Here's how the part is built. I have some questions about the finished solid (model axes, mm). A direction names the side the tool comes from. Coordinates: 2 decimals unless noted, no trailing zeros. Loops run counter-clockwise (first coordinate to the right, second up) from the corner with the lowest first, then second, coordinate; pieces in that order, holes last. Notation, with made-up numbers: (-18.5, -2.5) -> (34.5, -2.5) arc R23 ccw to (34.5, 7.5) -> close; hole circle Ø1 at (24.25, 3). An arc over 180 degrees is marked (long way). Answer as a JSON object with one key per item and string values. Group by question number.
1) Which directions (+Z, -Z, +X, -X, +Y, -Y) give clear straight access to the entire face, cutting with the end or side of a thin tool? Please do faces 4 (the flat face through (2, 141, 17)), 5 (the flat face through (-2, 278, 0)).
2) I want a section at A-A (z = 6.5). Write out the boundary of the cut face in (x, y), then the cut area to 3 significant figures.
3) I want a section at B-B (x = -34.5). Write out the boundary of the cut face in (y, z), then the cut area to 3 significant figures.
4) I need wall thicknesses on probe 1 along X at (y, z) = (82.5, 1); probe 2 along Y at (x, z) = (-96, 8); probe 3 along Y at (x, z) = (-36.5, -8). Which ranges of each line are inside material? Lowest first, please. Write a range as [from, to].
5) I want a section at C-C (y = 229). Write out the boundary of the cut face in (x, z).
6) I want a section at D-D (z = -11). Write out the boundary of the cut face in (x, y).
7) I'm going to push flat-ended pins straight in: pin 1 (2 mm diameter, centred on x = 19, y = 276, fed in from -Z); pin 2 (3 mm diameter, centred on x = -46.5, y = 73.5, fed in from -Z). Where does each tip first touch, or does it pass through?
8) If we mould it in two halves opening along Y, with no side actions, what happens to faces 1 (the flat face through (134, 137, 0)), 2 (the flat face through (2, 274, -1)), 3 (the flat face through (-2, 0, 0))? For each: +Y half, -Y half, draft (parallel to the pull), parting line (faces both ways), or undercut.
```python
from build123d import *

# Parameters (mm, degrees)
SKETCH_1_W          = 268
SKETCH_1_H          = 38
EXTRUDE_1_DEPTH     = 278
SKETCH_2_W          = 260
SKETCH_2_H          = 270
CUT_EXTRUDE_1_DEPTH = 36
CUT_EXTRUDE_2_REACH = 311.194
SKETCH_3_W          = 100
SKETCH_3_H          = 16
FILLET_1_R          = 2


with BuildPart() as part:
    # 草图1 → 凸台-拉伸1 (new body)
    with BuildSketch(Plane(origin=(0, 0, 0), x_dir=(1, 0, 0), z_dir=(0, 1, 0))):
        Rectangle(SKETCH_1_W, SKETCH_1_H)
    extrude(amount=EXTRUDE_1_DEPTH)

    # 草图2 → 切除-拉伸1 (cut)
    with BuildSketch(Plane(origin=(0, 0, -19), x_dir=(-1, 0, 0), z_dir=(0, 0, -1))):
        with Locations((0, 139)):
            Rectangle(SKETCH_2_W, SKETCH_2_H)
    extrude(amount=-CUT_EXTRUDE_1_DEPTH, mode=Mode.SUBTRACT)

    # 草图3 → 切除-拉伸2 (cut, up to next)
    with BuildSketch(Plane(origin=(0, 278, 0), x_dir=(1, 0, 0), z_dir=(0, 1, 0)), mode=Mode.PRIVATE) as cut_extrude_2_sk1:
        with Locations((0, 11)):
            Rectangle(SKETCH_3_W, SKETCH_3_H)
    cut_extrude_2_tool1 = extrude(cut_extrude_2_sk1.sketch, amount=-CUT_EXTRUDE_2_REACH, mode=Mode.PRIVATE) & part.part
    add(cut_extrude_2_tool1.solids().sort_by_distance((0, 278, -11))[0], mode=Mode.SUBTRACT)

    # 圆角1
    fillet_1_edges = [part.edges().sort_by_distance(p)[0] for p in [
        (134, 278, 0),
        (-50, 276, -3),
        (-50, 276, -19),
        (50, 276, -19),
        (50, 276, -3),
        (-134, 278, 0),
        (0, 0, -19),
        (134, 0, 0),
        (0, 0, 19),
        (-134, 0, 0),
        (-134, 139, -19),
        (134, 139, -19),
        (134, 139, 19),
        (-134, 139, 19),
    ]]
    fillet(fillet_1_edges, radius=FILLET_1_R)


solid = part.part
```
Determined:
{
 "1": {"face 4": "-Z", "face 5": "+Z, -Z, +X, -X, +Y"},
 "2": {"outline": "(-134, 2) arc R2 ccw to (-132, 0) -> (132, 0) arc R2 ccw to (134, 2) -> (134, 276) arc R2 ccw to (132, 278) -> (-132, 278) arc R2 ccw to (-134, 276) -> close; hole (-130, 4) -> (130, 4) -> (130, 274) -> (-130, 274) -> close", "area": "4,300 mm^2"},
 "3": {"outline": "(0, -17) arc R2 ccw to (2, -19) -> (4, -19) -> (4, 17) -> (274, 17) -> (274, -3) -> (278, -3) -> (278, 19) -> (2, 19) arc R2 ccw to (0, 17) -> close", "area": "778 mm^2"},
 "4": {"probe 1": "[-134, -130], [130, 134]", "probe 2": "[0, 4], [274, 278]", "probe 3": "[0, 4]"},
 "5": {"outline": "(-134, -17) arc R2 ccw to (-132, -19) -> (-130, -19) -> (-130, 17) -> (130, 17) -> (130, -19) -> (132, -19) arc R2 ccw to (134, -17) -> (134, 17) arc R2 ccw to (132, 19) -> (-132, 19) arc R2 ccw to (-134, 17) -> close"},
 "6": {"outline": "(-134, 2) arc R2 ccw to (-132, 0) -> (132, 0) arc R2 ccw to (134, 2) -> (134, 276) arc R2 ccw to (132, 278) -> (50, 278) -> (50, 274) -> (130, 274) -> (130, 4) -> (-130, 4) -> (-130, 274) -> (-50, 274) -> (-50, 278) -> (-132, 278) arc R2 ccw to (-134, 276) -> close"},
 "7": {"pin 1": "z = -3", "pin 2": "z = 17"},
 "8": {"face 1": "draft", "face 2": "undercut", "face 3": "-Y half"}
}
